Can you work these out from the model? Positions are in its coordinate system, mm. Face numbers are marked on the shaded views. Round coordinates to 2 decimals unless told otherwise and drop trailing zeros. Write each loop counter-clockwise with the first axis right and the second up, starting at its lowest first coordinate (ties: lowest second). Pieces come first, ordered by that corner, then holes. Notation, with made-up numbers: (57, -25.5) - (72, -25.5) arc R10 ccw to (72, -13.5) - close; hole circle Ø3 at (73.5, 3). An arc over 180 degrees is marked (long way). One line per item, written item: value. Start each with the question number.
(1) Thinking about a two-plate mould opening in Y: for the marked faces 1, 2 and 3, which applies, +Y half, -Y half, draft (parallel to the pull), parting line (faces both ways), or undercut?
(2) I want a section at A-A on y = 0. List the corners of the cut face in (x, z) for me.
(3) I want a section at C-C on z = 2.1. List the corners of the cut face in (x, y) for me, plus the area to 3 significant figures.
(4) I want a section at B-B on x = 0. List the corners of the cut face in (y, z) for me, plus the area to 3 significant figures.
(5) I'm going to push flat-ended pins straight in: pin 1 Ø3.5 at (x, y) = (0, 13) entering from +Z; pin 2 Ø1.5 at (x, z) = (2, 1) entering from -Y. Where does each tip first touch, or does it pass through?
(6) If I drill on L1, parallel to Y at x = 0, z = 1.8; L2, parallel to Y at x = 0.55, z = 2.7; L3, parallel to X at y = 1, z = 2.3, over which ranges is the centre line in solid material (lowest first)? Write a range as from..to.
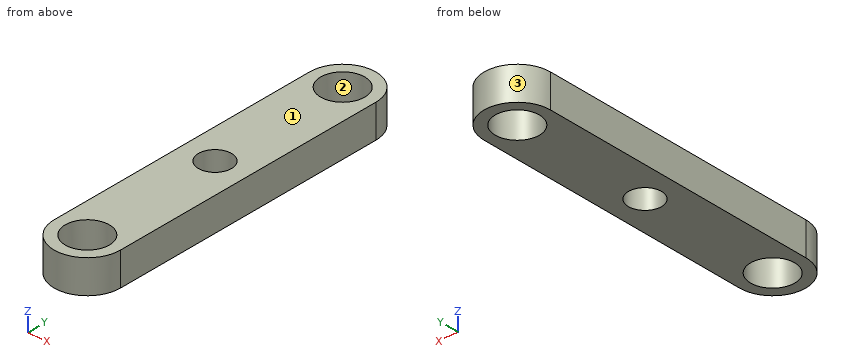
from build123d import *

# Parameters (mm, degrees)
SKETCH1_R           = 1.5
BOSS_EXTRUDE1_DEPTH = 3
SKETCH3_R           = 2
CUT_EXTRUDE2_DEPTH  = 10


with BuildPart() as part:
    # Sketch1 → Boss-Extrude1 (new body)
    with BuildSketch(Plane.XY):
        with BuildLine():
            Line((3, 13), (3, -13))
            ThreePointArc((3, -13), (0, -16), (-3, -13))
            Line((-3, -13), (-3, 13))
            ThreePointArc((-3, 13), (0, 16), (3, 13))
        make_face()
        with Locations((0, 13)):
            Circle(SKETCH1_R, mode=Mode.SUBTRACT)
        with Locations((0, -13)):
            Circle(SKETCH1_R, mode=Mode.SUBTRACT)
        Circle(SKETCH1_R, mode=Mode.SUBTRACT)
    extrude(amount=BOSS_EXTRUDE1_DEPTH)

    # Sketch3 → Cut-Extrude2 (cut)
    with BuildSketch(Plane.XY.offset(3)):
        with Locations((0, -13)):
            Circle(SKETCH3_R)
        with Locations((0, 13)):
            Circle(SKETCH3_R)
    extrude(amount=-CUT_EXTRUDE2_DEPTH, mode=Mode.SUBTRACT)


solid = part.part
Established:
1. face 1: draft
1. face 2: undercut
1. face 3: +Y half
2. outline: (-3, 0) - (-1.5, 0) - (-1.5, 3) - (-3, 3) - close; (1.5, 0) - (3, 0) - (3, 3) - (1.5, 3) - close
3. outline: (-3, -13) arc R3 ccw to (3, -13) - (3, 13) arc R3 ccw to (-3, 13) - close; hole circle Ø4 at (0, -13); hole circle Ø4 at (0, 13); hole circle Ø3 at (0, 0)
3. area: 152 mm2
4. outline: (-16, 0) - (-15, 0) - (-15, 3) - (-16, 3) - close; (-11, 0) - (-1.5, 0) - (-1.5, 3) - (-11, 3) - close; (1.5, 0) - (11, 0) - (11, 3) - (1.5, 3) - close; (15, 0) - (16, 0) - (16, 3) - (15, 3) - close
4. area: 63.0 mm2
5. pin 1: through
5. pin 2: y = -15.73
6. L1: -16..-15, -11..-1.5, 1.5..11, 15..16
6. L2: -15.95..-14.92, -11.08..-1.4, 1.4..11.08, 14.92..15.95
6. L3: -3..-1.12, 1.12..3
